Design review of the part built by this model. Coordinates are the model's own, in mm. Face numbers are marked on the shaded views. A direction names the side the tool comes from. Round coordinates to 2 decimals unless told otherwise and drop trailing zeros. Order: outer loops, then holes, each group sorted by start corner. A loop starts at its lowest first (then second) coordinate and runs counter-clockwise, first axis right, second up. Notation, with made-up numbers: (10.5, 61) - (63.5, 61) arc R19 cw to (63.5, 86) - close; hole circle Ø9 at (2.5, 57). An arc over 180 degrees is marked (long way). Use CSV: the item, a comma, the result in double quotes.
from build123d import *

# Parameters (mm, degrees)
SKETCH_1_W                  = 57.4
SKETCH_1_H                  = 28.5
EXTRUDE_1_DEPTH             = 12
SKETCH_2_W                  = 57.4
SKETCH_2_H                  = 26
EXTRUDE_2_DEPTH             = 19
SKETCH_3_W                  = 16.1
SKETCH_3_H                  = 20.5
CUT_EXTRUDE_1_DEPTH         = 7.7
SKETCH_4_W                  = 28.1
SKETCH_4_H                  = 20.5
CUT_EXTRUDE_2_DEPTH         = 41.7
SKETCH_5_W                  = 31
SKETCH_5_H                  = 20.5
CUT_EXTRUDE_3_DEPTH         = 0.3
CUT_EXTRUDE_4_DEPTH         = 2.9
SKETCH_7_W                  = 12
SKETCH_7_H                  = 2.5
CUT_EXTRUDE_5_DEPTH         = 46.4
CUT_EXTRUDE_6_DEPTH         = 7.7
CUT_EXTRUDE_7_DEPTH         = 14.1
CUT_EXTRUDE_8_DEPTH         = 3.3
SKETCH_11_W                 = 11
SKETCH_11_H                 = 12
EXTRUDE_3_DEPTH             = 2.5
SKETCH_12_W                 = 12
SKETCH_12_H                 = 2.75
EXTRUDE_4_DEPTH             = 6
SKETCH_13_W                 = 6
SKETCH_13_H                 = 12
EXTRUDE_5_DEPTH             = 2.5
SKETCH_14_W                 = 12
SKETCH_14_H                 = 5.25
EXTRUDE_6_DEPTH             = 6
SKETCH_15_W                 = 5
SKETCH_15_H                 = 2.5
CUT_EXTRUDE_9_DEPTH         = 45.999333328
SKETCH_16_W                 = 5
SKETCH_16_H                 = 2.5
CUT_EXTRUDE_10_DEPTH        = 45.999333328
SKETCH_17_W                 = 5
SKETCH_17_H                 = 26
EXTRUDE_7_DEPTH             = 2
SKETCH_19_W                 = 4
SKETCH_19_H                 = 6.5
HOLE_WIZARD_3_5_3_5_1_D     = 3.5
HOLE_WIZARD_3_5_3_5_1_DEPTH = 12
HOLE_WIZARD_3_0_3_3_D       = 3
HOLE_WIZARD_3_0_3_3_DEPTH   = 37.5
HOLE_WIZARD_3_5_3_5_3_D     = 3.5
FILLET_1_R                  = 7
EXTRUDE_START               = -19
SKETCH_28_W                 = 6
SKETCH_28_H                 = 5.25
SKETCH_28_R                 = 1.75
EXTRUDE_8_DEPTH             = 7


with BuildPart() as part:
    # Эскиз1 → Бобышка-Вытянуть1 (new body)
    with BuildSketch(Plane.XY.offset(12)):
        with Locations((0, 1.25)):
            Rectangle(SKETCH_1_W, SKETCH_1_H)
    extrude(amount=-EXTRUDE_1_DEPTH)

    # Эскиз2 → Бобышка-Вытянуть2 (add)
    with BuildSketch(Plane.XY.offset(12)):
        Rectangle(SKETCH_2_W, SKETCH_2_H)
    extrude(amount=EXTRUDE_2_DEPTH)

    # Эскиз3 → Вырез-Вытянуть1 (cut)
    with BuildSketch(Plane.ZY.offset(28.7)):
        with Locations((20.05, 0)):
            Rectangle(SKETCH_3_W, SKETCH_3_H)
    extrude(amount=-CUT_EXTRUDE_1_DEPTH, mode=Mode.SUBTRACT)

    # Эскиз4 → Вырез-Вытянуть2 (cut)
    with BuildSketch(Plane.ZY.offset(21)):
        with Locations((14.05, 0)):
            Rectangle(SKETCH_4_W, SKETCH_4_H)
    extrude(amount=-CUT_EXTRUDE_2_DEPTH, mode=Mode.SUBTRACT)

    # Эскиз5 → Вырез-Вытянуть3 (cut)
    with BuildSketch(Plane.ZY.offset(-20.7)):
        with Locations((15.5, 0)):
            Rectangle(SKETCH_5_W, SKETCH_5_H)
    extrude(amount=-CUT_EXTRUDE_3_DEPTH, mode=Mode.SUBTRACT)

    # Эскиз6 → Вырез-Вытянуть4 (cut)
    with BuildSketch(Plane.XY.offset(31)):
        Polygon((28.7, -13), (28.7, 13), (20.7, 13), (20.7, 10.25), (21, 10.25), (21, -10.25), (20.7, -10.25), (20.7, -13), align=None)
    extrude(amount=-CUT_EXTRUDE_4_DEPTH, mode=Mode.SUBTRACT)

    # Эскиз7 → Вырез-Вытянуть5 (cut)
    with BuildSketch(Plane(origin=(28.7, 0, 0), x_dir=(0, 0, -1), z_dir=(1, 0, 0))):
        with Locations((-6, 14.25)):
            Rectangle(SKETCH_7_W, SKETCH_7_H)
    extrude(amount=-CUT_EXTRUDE_5_DEPTH, mode=Mode.SUBTRACT)

    # Эскиз8 → Вырез-Вытянуть6 (cut)
    with BuildSketch(Plane.ZY.offset(28.7)):
        Polygon((12, -13), (31, -13), (31, 13), (12, 13), (12, 10.25), (28.1, 10.25), (28.1, -10.25), (12, -10.25), align=None)
    extrude(amount=-CUT_EXTRUDE_6_DEPTH, mode=Mode.SUBTRACT)

    # Эскиз9 → Вырез-Вытянуть7 (cut)
    with BuildSketch(Plane.XY.offset(28.1)):
        Polygon((28.7, -13), (28.7, 13), (20.7, 13), (20.7, 10.25), (21, 10.25), (21, -10.25), (20.7, -10.25), (20.7, -13), align=None)
    extrude(amount=-CUT_EXTRUDE_7_DEPTH, mode=Mode.SUBTRACT)

    # Эскиз10 → Вырез-Вытянуть8 (cut)
    with BuildSketch(Plane.ZY.offset(21)):
        Polygon((12, -13), (31, -13), (31, 13), (12, 13), (12, 10.25), (28.1, 10.25), (28.1, -10.25), (12, -10.25), align=None)
    extrude(amount=-CUT_EXTRUDE_8_DEPTH, mode=Mode.SUBTRACT)

    # Эскиз11 → Бобышка-Вытянуть3 (add)
    with BuildSketch(Plane.XZ.offset(13)):
        with Locations((-23.2, 6)):
            Rectangle(SKETCH_11_W, SKETCH_11_H)
    extrude(amount=EXTRUDE_3_DEPTH)

    # Эскиз12 → Бобышка-Вытянуть4 (add)
    with BuildSketch(Plane.ZY.offset(17.7)):
        with Locations((25, -11.625)):
            Rectangle(SKETCH_12_W, SKETCH_12_H)
    extrude(amount=EXTRUDE_4_DEPTH)

    # Эскиз13 → Бобышка-Вытянуть5 (add)
    with BuildSketch(Plane.XZ.offset(13)):
        with Locations((-20.7, 25)):
            Rectangle(SKETCH_13_W, SKETCH_13_H)
    extrude(amount=EXTRUDE_5_DEPTH)

    # Эскиз14 → Бобышка-Вытянуть6 (add)
    with BuildSketch(Plane.ZY.offset(17.7)):
        with Locations((25, 12.875)):
            Rectangle(SKETCH_14_W, SKETCH_14_H)
    extrude(amount=EXTRUDE_6_DEPTH)

    # Эскиз15 → Вырез-Вытянуть9 (cut, through all)
    with BuildSketch(Plane(origin=(0, 0, 0), x_dir=(-1, 0, 0), z_dir=(0, 0, -1))):
        with Locations((26.2, -14.25)):
            Rectangle(SKETCH_15_W, SKETCH_15_H)
    extrude(amount=-CUT_EXTRUDE_9_DEPTH, mode=Mode.SUBTRACT)

    # Эскиз16 → Вырез-Вытянуть10 (cut, through all)
    with BuildSketch(Plane(origin=(0, 0, 0), x_dir=(-1, 0, 0), z_dir=(0, 0, -1))):
        with Locations((26.2, 14.25)):
            Rectangle(SKETCH_16_W, SKETCH_16_H)
    extrude(amount=-CUT_EXTRUDE_10_DEPTH, mode=Mode.SUBTRACT)

    # Эскиз17 → Бобышка-Вытянуть7 (add)
    with BuildSketch(Plane.XY.offset(12)):
        with Locations((-26.2, 0)):
            Rectangle(SKETCH_17_W, SKETCH_17_H)
    extrude(amount=EXTRUDE_7_DEPTH)

    # Эскиз19 → Повернуть1 (revolve)
    with BuildSketch(Plane.XZ, mode=Mode.PRIVATE) as revolve_1_sk:
        with Locations((12.2, 34.25)):
            Rectangle(SKETCH_19_W, SKETCH_19_H)
    revolve(revolve_1_sk.sketch.rotate(Axis((10.2, 0, 37.5), (0, 0, -1)), 180), axis=Axis((10.2, 0, 37.5), (0, 0, -1)))

    # Диаметр отверстия Ø3.5 (3.5)1
    with Locations(Plane.XY.offset(31)):
        with Locations((-20.7, 13), (-20.7, -13)):
            Hole(HOLE_WIZARD_3_5_3_5_1_D / 2, depth=HOLE_WIZARD_3_5_3_5_1_DEPTH)

    # Диаметр отверстия Ø3.0 (3)3
    with Locations(Plane(origin=(0, 0, 0), x_dir=(-1, 0, 0), z_dir=(0, 0, -1))):
        with Locations((-25.5, -5), (-25.5, 5), (25.5, -5), (25.5, 5)):
            Hole(HOLE_WIZARD_3_0_3_3_D / 2, depth=HOLE_WIZARD_3_0_3_3_DEPTH)

    # Диаметр отверстия Ø3.5 (3.5)3 (through all)
    with Locations(Plane.XY.offset(12)):
        with Locations((-20.7, 13), (-20.7, -13)):
            Hole(HOLE_WIZARD_3_5_3_5_3_D / 2)

    # Скругление1
    fillet_1_edges = [part.edges().sort_by_distance(p)[0] for p in [
        (28.7, 13, 7),
        (28.7, -13, 7),
    ]]
    fillet(fillet_1_edges, radius=FILLET_1_R)

    # Эскиз28 → Бобышка-Вытянуть8 (add)
    # profile 1 of 2: a face of its own
    with BuildSketch(Plane.XY.offset(31).offset(EXTRUDE_START)):
        with Locations((-20.7, 12.875)):
            Rectangle(SKETCH_28_W, SKETCH_28_H)
        with Locations((-20.7, 13)):
            Circle(SKETCH_28_R, mode=Mode.SUBTRACT)
    # profile 2 of 2: a face of its own
    with BuildSketch(Plane.XY.offset(31).offset(EXTRUDE_START)):
        with Locations((-20.7, -12.875)):
            Rectangle(SKETCH_28_W, SKETCH_28_H)
        with Locations((-20.7, -13)):
            Circle(SKETCH_28_R, mode=Mode.SUBTRACT)
    extrude(amount=EXTRUDE_8_DEPTH)


solid = part.part
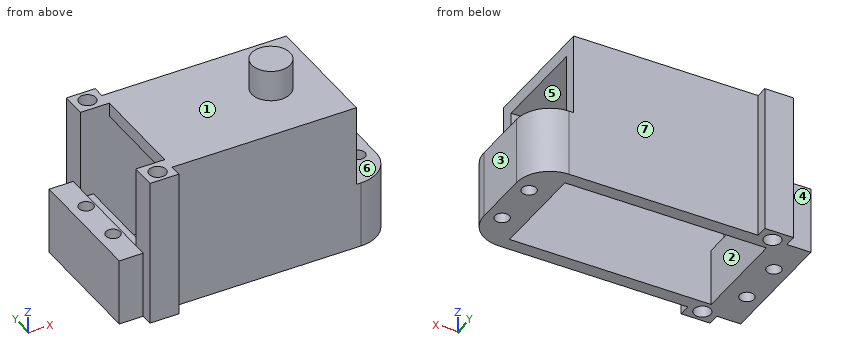
1) We need section A-A (z = 24). Give the boundary of the cut face in (x, y).
Data:
outline,"(-23.7, -15.5) - (-17.7, -15.5) - (-17.7, -13) - (20.7, -13) - (20.7, -10.25) - (-23.7, -10.25) - close; (-23.7, 10.25) - (20.7, 10.25) - (20.7, 13) - (-17.7, 13) - (-17.7, 15.5) - (-23.7, 15.5) - close; hole circle Ø3.5 at (-20.7, -13); hole circle Ø3.5 at (-20.7, 13)"
2) To check wall thickness, follow L1, parallel to Y at x = 17.5, z = 20.5; L2, parallel to Y at x = 25, z = 10; L3, parallel to Y at x = 25.5, z = 8.75. State the ranges of each line that lie inside material, in increasing order. Write a range as from..to.
Data:
L1,"y = -13..-10.25, 10.25..13"
L2,"y = -12.17..-6.41, -3.59..3.59, 6.41..12.17"
L3,"y = -11.88..-6.5, -3.5..3.5, 6.5..11.88"
3) We need section D-D (x = 25.5). Give the boundary of the cut face in (y, z).
Data:
outline,"(-11.88, 0) - (-6.5, 0) - (-6.5, 14) - (-11.88, 14) - close; (-3.5, 0) - (3.5, 0) - (3.5, 14) - (-3.5, 14) - close; (6.5, 0) - (11.88, 0) - (11.88, 14) - (6.5, 14) - close"
4) The part is to be moulded in two halves that separate along X. For the marked faces 1, 2 and 3, say which applies: +X half, -X half, draft (parallel to the pull), parting line (faces both ways), or undercut.
Data:
face 1,"draft"
face 2,"undercut"
face 3,"+X half"
5) Insertion check: pin 1 Ø4 at (x, y) = (-25.5, -5) entering from -Z; pin 2 Ø5 at (x, z) = (3, 30.5) entering from -Y; pin 3 Ø3 at (x, y) = (-20.7, 13) entering from +Z; pin 4 Ø5 at (x, z) = (-7, 15) entering from +Y. Each pin has a flat end and moves straight along its axis. Give the tip position at first contact, or say it passes through.
Data:
pin 1,"stops at z = 0"
pin 2,"stops at y = -13"
pin 3,"passes through"
pin 4,"stops at y = 13"
6) For the marked faces 4, 5, 6 and 7, list the 3-axis set-ups (+Z, -Z, +X, -X, +Y, -Y) from which the entire face can be reached by the end or side of a thin tool; tool diameter is ignored.
Data:
face 4,"+Z, -Z, -X, +Y"
face 5,"-Z, +X, -X"
face 6,"+Z, +X, +Y, -Y"
face 7,"+Z, -Z, +X, +Y"
7) We need section B-B (y = -8). Give the boundary of the cut face in (x, z).
Data:
outline,"(-28.7, 0) - (-21, 0) - (-21, 12) - (-23.7, 12) - (-23.7, 14) - (-28.7, 14) - close; (-17.7, 28.1) - (20.7, 28.1) - (20.7, 31) - (-17.7, 31) - close; (21, 0) - (28.41, 0) - (28.41, 14) - (21, 14) - close"
8) We need section C-C (x = -7). Give the boundary of the cut face in (y, z), then the cut area to 3 significant figures.
Data:
outline,"(-13, 0) - (-10.25, 0) - (-10.25, 28.1) - (10.25, 28.1) - (10.25, 0) - (13, 0) - (13, 31) - (-13, 31) - close"
area,"230 mm2"
